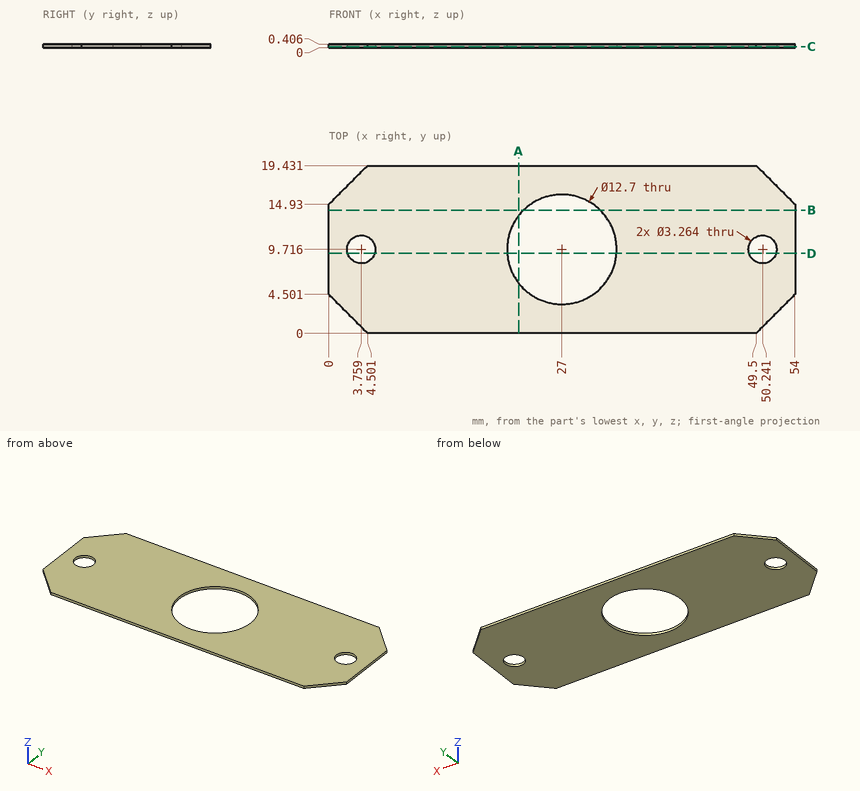
Check sheet for the drawn part. Datum: minimum x, y, z corner. Units: mm. Give positions to 0.01 mm unless a question says otherwise; leave off trailing zeros. Order: outer loops, then holes, each group sorted by start corner. A loop starts at its lowest first (then second) coordinate and runs counter-clockwise, first axis right, second up. Notation, with made-up numbers: (18, 45.25) -> (35, 45.25) arc R23 cw to (35, 61.25) -> close; hole circle Ø1 at (-30.75, -7.75). An arc over 180 degrees is marked (long way). One line per item, written item: value.
(1) Sectioned sample at D-D on y = 9.25. Record the cut outline in (x, z) (1 decimal).
Final values:
outline: (0, 0) -> (2.2, 0) -> (2.2, 0.4) -> (0, 0.4) -> close; (5.3, 0) -> (20.7, 0) -> (20.7, 0.4) -> (5.3, 0.4) -> close; (33.3, 0) -> (48.7, 0) -> (48.7, 0.4) -> (33.3, 0.4) -> close; (51.8, 0) -> (54, 0) -> (54, 0.4) -> (51.8, 0.4) -> close
(2) Sectioned sample at A-A on x = 22. Record the cut outline in (y, z).
Final values:
outline: (0, 0) -> (5.8, 0) -> (5.8, 0.41) -> (0, 0.41) -> close; (13.63, 0) -> (19.43, 0) -> (19.43, 0.41) -> (13.63, 0.41) -> close
(3) Sectioned sample at B-B on y = 14.25. Record the cut outline in (x, z) (1 decimal).
Final values:
outline: (0, 0) -> (22.6, 0) -> (22.6, 0.4) -> (0, 0.4) -> close; (31.4, 0) -> (54, 0) -> (54, 0.4) -> (31.4, 0.4) -> close
(4) Scan lines: line 1 along X through (y, z) = (10.5, 0.15); line 2 along X through (y, z) = (8.75, 0.1) (1 decimal); line 3 along Y through (x, z) = (4, 0.15). Record each from-to range of solid material in increasing order. Write a range as [from, to].
Final values:
line 1: [0, 2.33], [5.19, 20.7], [33.3, 48.81], [51.67, 54]
line 2: [0, 2.4], [5.1, 20.7], [33.3, 48.9], [51.6, 54]
line 3: [0.5, 8.1], [11.33, 18.93]
(5) Gauge pin test, flat end, axial feed: pin 1 (1.5 mm diameter, centred on x = 30, y = 13.5, fed in from -Z). Record the tip position at first contact, or that the pin passes through.
Final values:
pin 1: through
(6) Sectioned sample at C-C on z = 0.1. Count the separate pieces of the cut face and the enclosed holes in it.
Final values:
separate pieces: 1
enclosed holes: 3
